The listing builds one solid part. Answer for the finished solid, in the listing's coordinates (mm). Give positions to 0.01 mm unless a question says otherwise; leave off trailing zeros. Order: outer loops, then holes, each group sorted by start corner. A loop starts at its lowest first (then second) coordinate and runs counter-clockwise, first axis right, second up. Notation, with made-up numbers: (-1.5, 52) - (53.5, 52) arc R23 cw to (53.5, 66) - close; hole circle Ø2 at (3.25, 20.25). An arc over 180 degrees is marked (long way). Write each question's results on one line, items separated by ' | '. Start each with the question number.
1. Find the intervals of material crossed by L1, parallel to Z at x = 135, y = 11; L2, parallel to Z at x = 221.5, y = 19.5; L3, parallel to X at y = 8, z = 11, in increasing order.
2. Section C-C (z = 3) is taken. Give the vertices of the cut face in (x, y), and give its area (3 significant figures).
3. Flat-ended cylindrical pins translate along their axes: pin 1 (2 mm diameter, centred on y = 8.5, z = 34, fed in from +X); pin 2 (3 mm diameter, centred on x = 80, y = 4.5, fed in from +Z). Find the tip coordinate at first contact, or state that the pin passes through.
4. Section A-A (y = 36.5) is taken. Give the vertices of the cut face in (x, z), and give its area (3 significant figures).
5. Section B-B (x = 205) is taken. Give the vertices of the cut face in (y, z).
from build123d import *

# Parameters (mm, degrees)
F1_DEPTH = 44.45
F3_DEPTH = 50.8


with BuildPart() as f1:
    # F0 (on Front) → F1 (new body)
    with BuildSketch(Plane.XZ):
        Polygon((0, 69.85), (0, 0), (304.8, 0), (304.8, 19.05), align=None)
    extrude(amount=-F1_DEPTH)

    # F2 (on face) → F3 (cut)
    with BuildSketch(Plane.XZ):
        with BuildLine():
            ThreePointArc((0, 45.065515), (39.269991, 43.781798), (76.421015, 30.991899))
            ThreePointArc((76.421015, 30.991899), (131.267893, 19.381868), (186.913863, 26.200881))
            ThreePointArc((186.913863, 26.200881), (247.918131, 22.374434), (304.8, 0))
            Line((304.8, 0), (304.8, 19.05))
            Line((304.8, 19.05), (0, 69.85))
            Line((0, 69.85), (0, 45.065515))
        make_face()
    extrude(amount=-F3_DEPTH, mode=Mode.SUBTRACT)


solid = f1.part
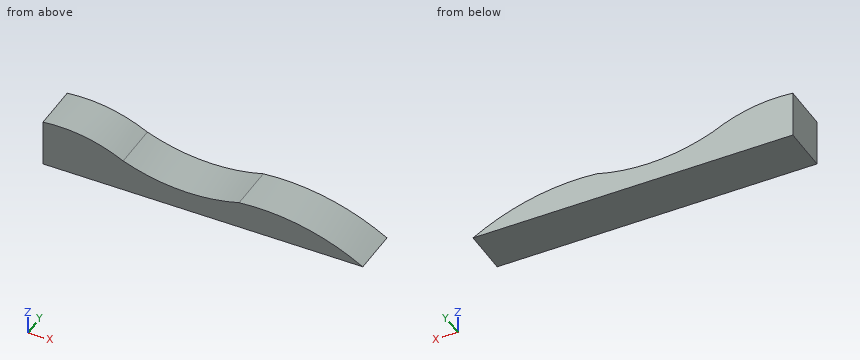
Reported:
1) L1: 0 to 19.26 | L2: 0 to 26.39 | L3: 0 to 283.08
2) outline: (0, 0) - (299.5, 0) - (299.5, 44.45) - (0, 44.45) - close | area: 13,300 mm²
3) pin 1: x = 72.41 | pin 2: z = 30.19
4) outline: (0, 0) - (304.8, 0) arc R196.63 ccw to (186.91, 26.2) arc R170.38 cw to (76.42, 30.99) arc R131.95 ccw to (0, 45.07) - close | area: 8,000 mm²
5) outline: (0, 0) - (44.45, 0) - (44.45, 27.06) - (0, 27.06) - close
